Check sheet for the modelled part. Datum: model origin and axes. Units: mm. Face numbers are marked on the shaded views. A direction names the side the tool comes from. Round coordinates to 2 decimals unless told otherwise and drop trailing zeros. Loops run counter-clockwise (first coordinate to the right, second up) from the corner with the lowest first, then second, coordinate; pieces in that order, holes last. Notation, with made-up numbers: (74, 65.5) -> (91, 65.5) arc R3 ccw to (91, 70.5) -> close; hole circle Ø10 at (27.25, -27). An arc over 180 degrees is marked (long way). Return JSON: item names as keys, results as strings.
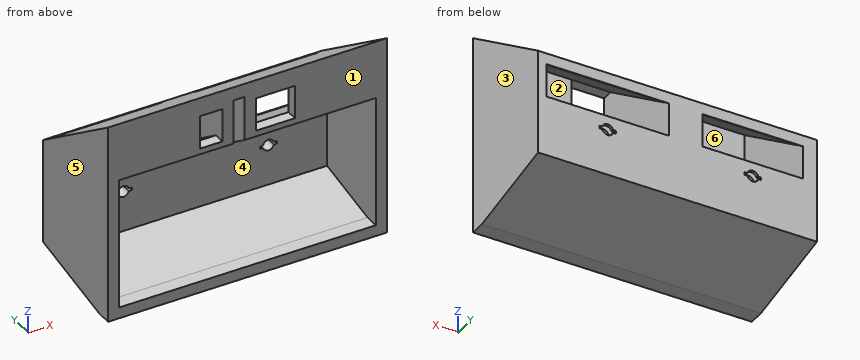
from build123d import *

# Parameters (mm, degrees)
SKIZZE1_W                            = 50
SKIZZE1_H                            = 30
AUFSATZ_LINEAR_AUSTRAGEN1_DEPTH      = 40
FPV_SENDER_START                     = -1.5
FPV_SENDER_DEPTH                     = 22
EMPF_NGER_START                      = 4.5
EMPF_NGER_DEPTH                      = 18
SCHNITT_LINEAR_AUSTRAGEN3_DEPTH      = 66.76473219
SCHNITT_LINEAR_AUSTRAGEN3_DEPTH_BACK = 66.76473219
SCHNITT_LINEAR_AUSTRAGEN5_REACH      = 65.411
WANDUNG2_START                       = -23
WANDUNG2_DEPTH                       = 46
WANDUNG2_START_2                     = -2.5
WANDUNG2_2_DEPTH                     = 2
SKIZZE6_W                            = 7
SKIZZE6_H                            = 6
SCHNITT_LINEAR_AUSTRAGEN4_DEPTH      = 2
SKIZZE8_W                            = 4
SKIZZE8_H                            = 6
SCHNITT_LINEAR_AUSTRAGEN7_DEPTH      = 2
SCHNITT_LINEAR_START                 = -2.5
SCHNITT_LINEAR_AUSTRAGEN8_DEPTH      = 18
SCHNITT_LINEAR_START_2               = -1.5
SCHNITT_LINEAR_AUSTRAGEN9_DEPTH      = 22
AUFSATZ_LINEAR_AUSTRAGEN2_REACH      = 63.847
SCHNITT_LINEAR_AUSTRAGEN10_REACH     = 50.177
SKIZZE11_R                           = 1
SKIZZE11_W                           = 3
SKIZZE11_H                           = 0.5


# Read off the part's stored shape, not the designer's step: Wandung2
with BuildPart() as part:
    # Skizze1 → Aufsatz-Linear austragen1 (new body)
    with BuildSketch(Plane.XY):
        Rectangle(SKIZZE1_W, SKIZZE1_H)
    extrude(amount=AUFSATZ_LINEAR_AUSTRAGEN1_DEPTH)

    # Skizze2 → FPV_Sender (cut)
    with BuildSketch(Plane.ZY.offset(FPV_SENDER_START)):
        Polygon((13.5, 15), (7.5, 15), (26.633333333, -13), (32.633333333, -13), align=None)
    extrude(amount=-FPV_SENDER_DEPTH, mode=Mode.SUBTRACT)

    # Skizze4 → Empfänger (cut)
    with BuildSketch(Plane.ZY.offset(EMPF_NGER_START)):
        Polygon((13.5, 15), (7.5, 15), (26.633333333, -13), (32.633333333, -13), align=None)
    extrude(amount=EMPF_NGER_DEPTH, mode=Mode.SUBTRACT)

    # Skizze5 → Schnitt-Linear austragen3 (cut, two sides: drawn at the far end of the back side and taken through both)
    with BuildSketch(Plane.ZY.offset(25).offset(-SCHNITT_LINEAR_AUSTRAGEN3_DEPTH_BACK)):
        Polygon((15.5, 15), (40, 15), (40, -20.853658537), align=None)
        Polygon((5.5, 15), (0, -12.25), (0, 15), align=None)
    extrude(amount=SCHNITT_LINEAR_AUSTRAGEN3_DEPTH + SCHNITT_LINEAR_AUSTRAGEN3_DEPTH_BACK, mode=Mode.SUBTRACT)

    # Schnitt-Linear austragen5: up to this face of the body (flat: up to its plane)
    schnitt_linear_austragen5_end = Plane(part.part.faces().sort_by_distance((-25, -2.83971717, 14.814249022))[0])
    # Skizze7 → Schnitt-Linear austragen5 (cut, up to the picked face)
    with BuildSketch(Plane(origin=(25, 0, 0), x_dir=(0, 0, -1), z_dir=(1, 0, 0)), mode=Mode.PRIVATE) as schnitt_linear_austragen5_sk1:
        Polygon((-5.5, 15), (-15.5, 15), (-22.333333333, 5), (-3.481651376, 5), align=None)
    schnitt_linear_austragen5_tool1 = split(extrude(schnitt_linear_austragen5_sk1.sketch, amount=-SCHNITT_LINEAR_AUSTRAGEN5_REACH, mode=Mode.PRIVATE), bisect_by=schnitt_linear_austragen5_end, keep=Keep.BOTH, mode=Mode.PRIVATE)
    add(schnitt_linear_austragen5_tool1.solids().sort_by(Axis((25, 9.488667, 11.826849), (-1, 0, 0)))[0], mode=Mode.SUBTRACT)

    # Wandung2 outline → Wandung2 (cut)
    with BuildSketch(Plane.YZ.offset(WANDUNG2_START)):
        Polygon((3, 13.27765036), (-15, 25.57765036), (-15, 2), (-12.449820142, 2), (3, 5.118312322), align=None)
    extrude(amount=WANDUNG2_DEPTH, mode=Mode.SUBTRACT)

    # Wandung2 2 outline → Wandung2 2 (cut)
    with BuildSketch(Plane.YZ.offset(WANDUNG2_START_2)):
        Polygon((-15, 33.57765036), (-15, 25.57765036), (3, 13.27765036), (3, 21.27765036), align=None)
    extrude(amount=WANDUNG2_2_DEPTH, mode=Mode.SUBTRACT)

    # Skizze6 → Schnitt-Linear austragen4 (cut)
    with BuildSketch(Plane(origin=(0, -13, 0), x_dir=(1, 0, 0), z_dir=(0, 1, 0))):
        with Locations((5, -29.633333333)):
            Rectangle(SKIZZE6_W, SKIZZE6_H)
    extrude(amount=-SCHNITT_LINEAR_AUSTRAGEN4_DEPTH, mode=Mode.SUBTRACT)

    # Skizze8 → Schnitt-Linear austragen7 (cut)
    with BuildSketch(Plane(origin=(0, -13, 0), x_dir=(1, 0, 0), z_dir=(0, 1, 0))):
        with Locations((-6.5, -29.633333333)):
            Rectangle(SKIZZE8_W, SKIZZE8_H)
    extrude(amount=-SCHNITT_LINEAR_AUSTRAGEN7_DEPTH, mode=Mode.SUBTRACT)

    # Skizze9 → Schnitt-Linear austragen8 (cut)
    with BuildSketch(Plane.ZY.offset(25).offset(SCHNITT_LINEAR_START)):
        Polygon((22.675, 4.5), (7.675, 4.5), (7.675, 3.5), (23.358333333, 3.5), align=None)
    extrude(amount=-SCHNITT_LINEAR_AUSTRAGEN8_DEPTH, mode=Mode.SUBTRACT)

    # Skizze10 → Schnitt-Linear austragen9 (cut)
    with BuildSketch(Plane(origin=(25, 0, 0), x_dir=(0, 0, -1), z_dir=(1, 0, 0)).offset(SCHNITT_LINEAR_START_2)):
        Polygon((-22.675, 4.5), (-7.675, 4.5), (-7.675, 3.5), (-23.358333333, 3.5), align=None)
    extrude(amount=-SCHNITT_LINEAR_AUSTRAGEN9_DEPTH, mode=Mode.SUBTRACT)

    # Aufsatz-Linear austragen2: up to this face of the body (flat: up to its plane)
    aufsatz_linear_austragen2_end = Plane(part.part.faces().sort_by_distance((23, -7.466953152, 11.743949806))[0])
    # Skizze12 → Aufsatz-Linear austragen2 (add, up to the picked face)
    with BuildSketch(Plane(origin=(-23, 0, 0), x_dir=(0, 0, -1), z_dir=(1, 0, 0)), mode=Mode.PRIVATE) as aufsatz_linear_austragen2_sk1:
        Polygon((-5.118312322, 3), (-13.27765036, 3), (-15.32765036, 0), (-4.512807735, 0), align=None)
    aufsatz_linear_austragen2_tool1 = split(extrude(aufsatz_linear_austragen2_sk1.sketch, amount=AUFSATZ_LINEAR_AUSTRAGEN2_REACH, mode=Mode.PRIVATE), bisect_by=aufsatz_linear_austragen2_end, keep=Keep.BOTH, mode=Mode.PRIVATE)
    add(aufsatz_linear_austragen2_tool1.solids().sort_by(Axis((-23, 1.430023, 9.575952), (1, 0, 0)))[0])

    # Schnitt-Linear austragen10: up to this face of the body (flat: up to its plane)
    schnitt_linear_austragen10_end = Plane(part.part.faces().sort_by_distance((0, 0, 9.920229048))[0])
    # Skizze11 → Schnitt-Linear austragen10 (cut, up to the picked face)
    with BuildSketch(Plane(origin=(0, 5, 0), x_dir=(1, 0, 0), z_dir=(0, 1, 0)), mode=Mode.PRIVATE) as schnitt_linear_austragen10_sk1:
        with Locations((12.5, -11.833333333)):
            Circle(SKIZZE11_R)
    schnitt_linear_austragen10_tool1 = split(extrude(schnitt_linear_austragen10_sk1.sketch, amount=-SCHNITT_LINEAR_AUSTRAGEN10_REACH, mode=Mode.PRIVATE), bisect_by=schnitt_linear_austragen10_end, keep=Keep.BOTH, mode=Mode.PRIVATE)
    # Skizze11 → Schnitt-Linear austragen10 (cut, up to the picked face)
    with BuildSketch(Plane(origin=(0, 5, 0), x_dir=(1, 0, 0), z_dir=(0, 1, 0)), mode=Mode.PRIVATE) as schnitt_linear_austragen10_sk2:
        with Locations((-13.5, -11.833333333)):
            Circle(SKIZZE11_R)
    schnitt_linear_austragen10_tool2 = split(extrude(schnitt_linear_austragen10_sk2.sketch, amount=-SCHNITT_LINEAR_AUSTRAGEN10_REACH, mode=Mode.PRIVATE), bisect_by=schnitt_linear_austragen10_end, keep=Keep.BOTH, mode=Mode.PRIVATE)
    # Skizze11 → Schnitt-Linear austragen10 (cut, up to the picked face)
    with BuildSketch(Plane(origin=(0, 5, 0), x_dir=(1, 0, 0), z_dir=(0, 1, 0)), mode=Mode.PRIVATE) as schnitt_linear_austragen10_sk3:
        with Locations((12.5, -11.833333333)):
            Rectangle(SKIZZE11_W, SKIZZE11_H)
    schnitt_linear_austragen10_tool3 = split(extrude(schnitt_linear_austragen10_sk3.sketch, amount=-SCHNITT_LINEAR_AUSTRAGEN10_REACH, mode=Mode.PRIVATE), bisect_by=schnitt_linear_austragen10_end, keep=Keep.BOTH, mode=Mode.PRIVATE)
    # Skizze11 → Schnitt-Linear austragen10 (cut, up to the picked face)
    with BuildSketch(Plane(origin=(0, 5, 0), x_dir=(1, 0, 0), z_dir=(0, 1, 0)), mode=Mode.PRIVATE) as schnitt_linear_austragen10_sk4:
        with Locations((-13.5, -11.833333333)):
            Rectangle(SKIZZE11_W, SKIZZE11_H)
    schnitt_linear_austragen10_tool4 = split(extrude(schnitt_linear_austragen10_sk4.sketch, amount=-SCHNITT_LINEAR_AUSTRAGEN10_REACH, mode=Mode.PRIVATE), bisect_by=schnitt_linear_austragen10_end, keep=Keep.BOTH, mode=Mode.PRIVATE)
    add(schnitt_linear_austragen10_tool1.solids().sort_by(Axis((12.5, 5, 11.833333), (0, -1, 0)))[0], mode=Mode.SUBTRACT)
    add(schnitt_linear_austragen10_tool2.solids().sort_by(Axis((-13.5, 5, 11.833333), (0, -1, 0)))[0], mode=Mode.SUBTRACT)
    add(schnitt_linear_austragen10_tool3.solids().sort_by(Axis((12.5, 5, 11.833333), (0, -1, 0)))[0], mode=Mode.SUBTRACT)
    add(schnitt_linear_austragen10_tool4.solids().sort_by(Axis((-13.5, 5, 11.833333), (0, -1, 0)))[0], mode=Mode.SUBTRACT)


solid = part.part
Q1. Draft check along X on the marked faces 1, 2 and 3. Enter one of: released by +X, released by -X, zero draft, split by the parting line, or undercut.
Results list:
{"face 1": "zero draft", "face 2": "undercut", "face 3": "released by +X"}
Q2. Material ranges on line 1 (X direction, y = -7.25, z = 25.5); line 2 (Z direction, x = -7.5, y = -11.75); line 3 (X direction, y = -11, z = 4.5), recorded low to high.
Results list:
{"line 1": "-25 to -22.5, -4.5 to -2.5, -0.5 to 1.5, 23.5 to 25", "line 2": "0.1 to 2.14, 23.36 to 25.78, 31.78 to 33.78", "line 3": "-25 to -23, 23 to 25"}
Q3. Section check C-C (x = -6.5). Record the boundary of the cut face in (y, z) (3 decimals), then the cut area to 3 significant figures.
Results list:
{"outline": "(-15, 0) -> (-12.25, 0) -> (5, 3.482) -> (5, 14.333) -> (4.5, 14.675) -> (4.5, 7.675) -> (3.5, 7.675) -> (3.5, 15.358) -> (-13, 26.633) -> (-15, 26.633) -> (-15, 25.578) -> (0, 15.328) -> (0, 4.513) -> (-12.45, 2) -> (-15, 2) -> close; (-15, 32.633) -> (-13, 32.633) -> (3.5, 21.358) -> (3.5, 23.358) -> (-15, 36) -> close; (4.5, 20.675) -> (5, 20.333) -> (5, 22.333) -> (4.5, 22.675) -> close", "area": "163 mm^2"}
Q4. Section check A-A (x = -20.5). Record the boundary of the cut face in (y, z) (3 decimals).
Results list:
{"outline": "(-15, 0) -> (-12.25, 0) -> (5, 3.482) -> (5, 14.333) -> (4.5, 14.675) -> (4.5, 7.675) -> (3.5, 7.675) -> (3.5, 15.358) -> (-13, 26.633) -> (-13, 32.633) -> (3.5, 21.358) -> (3.5, 23.358) -> (-15, 36) -> (-15, 25.578) -> (0, 15.328) -> (0, 4.513) -> (-12.45, 2) -> (-15, 2) -> close; (4.5, 20.675) -> (5, 20.333) -> (5, 22.333) -> (4.5, 22.675) -> close"}
Q5. Section check B-B (y = -10.75). Record the boundary of the cut face in (x, z), then the cut area to 3 significant figures.
Results list:
{"outline": "(-25, 0.3) -> (25, 0.3) -> (25, 33.1) -> (-25, 33.1) -> close; hole (-23, 2.34) -> (23, 2.34) -> (23, 22.67) -> (-0.5, 22.67) -> (-0.5, 30.67) -> (-2.5, 30.67) -> (-2.5, 22.67) -> (-23, 22.67) -> close; hole (-22.5, 25.1) -> (-4.5, 25.1) -> (-4.5, 31.1) -> (-22.5, 31.1) -> close; hole (1.5, 25.1) -> (23.5, 25.1) -> (23.5, 31.1) -> (1.5, 31.1) -> close", "area": "448 mm^2"}
Q6. Go/stop test with flat-tipped pins: pin 1 (3 mm diameter, centred on x = 2, z = 15, fed in from -Y); pin 2 (2 mm diameter, centred on x = 16, y = 2, fed in from -Z); pin 3 (4 mm diameter, centred on x = 9.5, y = -4, fed in from -Z). Record where each tip stops, or that it passes through.
Results list:
{"pin 1": "y = -1.72", "pin 2": "z = 2.67", "pin 3": "z = 1.26"}
Q7. Tool access check on the marked faces 4, 5 and 6. Record the directions out of +Z, -Z, +X, -X, +Y, -Y that give a thin tool (end or side, any length) a straight path to the whole face; none if there is none.
Results list:
{"face 4": "-Y", "face 5": "+Z, -Z, -X, +Y, -Y", "face 6": "none"}
Q8. Section check D-D (z = 28.5). Record the boundary of the cut face in (x, y).
Results list:
{"outline": "(-25, -15) -> (-8.5, -15) -> (-8.5, -13) -> (-22.5, -13) -> (-22.5, -6.95) -> (-4.5, -6.95) -> (-4.5, -15) -> (-2.5, -15) -> (-2.5, -7.57) -> (-0.5, -7.57) -> (-0.5, -15) -> (1.5, -15) -> (1.5, -6.95) -> (23.5, -6.95) -> (23.5, -13) -> (8.5, -13) -> (8.5, -15) -> (25, -15) -> (25, -4.02) -> (-25, -4.02) -> close"}
